Design review of the part built by this model. Coordinates are the model's own, in mm. Face numbers are marked on the shaded views. A direction names the side the tool comes from. Round coordinates to 2 decimals unless told otherwise and drop trailing zeros. Write each loop counter-clockwise with the first axis right and the second up, starting at its lowest first coordinate (ties: lowest second). Pieces come first, ordered by that corner, then holes. Notation, with made-up numbers: (-24.75, 27.25) -> (32.25, 27.25) arc R14 cw to (32.25, 50.25) -> close; hole circle Ø3 at (17, -33.75). An arc over 180 degrees is marked (long way). Write item = value, one per line. Start each with the question number.
Item 1: Machinability: for the marked faces 4 and 5, which of the approach directions +Z, -Z, +X, -X, +Y, -Y give a long, thin tool a straight path to every point of the face, cutting with its end or side? Answer none if there is none.
Item 2: For pin 1 Ø4.5 at (x, y) = (-20, 7) entering from +Z; pin 2 Ø1.2 at (x, z) = (0, 11.5) entering from -Y; pin 3 Ø1.2 at (x, y) = (-20, -6) entering from +Z; pin 4 Ø1.8 at (x, y) = (20.59, 6.89) entering from +Z, all flat-tipped, find the tip position at first contact; note any pin that passes through.
Item 3: Add section D-D, the plane y = -1.25. State the section outline as (x, z) points.
Item 4: Add section C-C, the plane x = -14.5. State the section outline as (y, z) points, then the cut area to 3 significant figures.
Item 5: To check wall thickness, follow L1, parallel to Y at x = -20.59, z = 0.45; L2, parallel to Z at x = 0, y = -14.3 (3 decimals); L3, parallel to Y at x = -17, z = 11.75. State the ranges of each line that lie inside material, in increasing order.
Item 6: Add section A-A, the plane x = -20.59. State the section outline as (y, z) points.
Item 7: Add section B-B, the plane z = 11.1. State the section outline as (x, y) points (3 decimals).
Item 8: Mouldability with a two-part tool opening along X and no side actions: class the marked faces 1, 2 and 3 as released by +X, released by -X, zero draft, split by the parting line, or undercut.
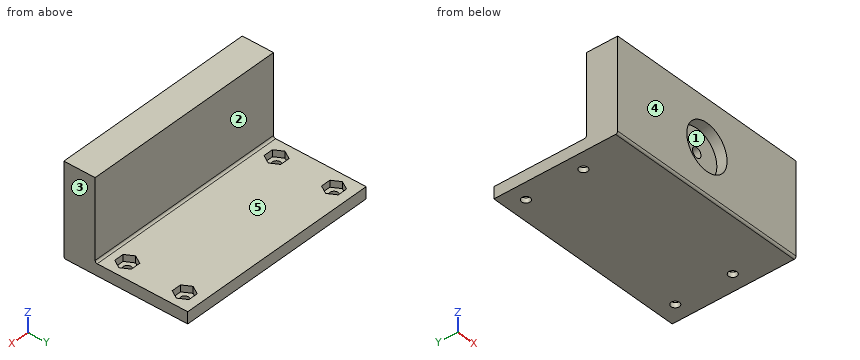
Autodesk Fusion 360 part; units mm, degrees
sketch "Boceto1" plane through (0, 0, 0) normal (0, 0, 1) x (1, 0, 0)
  line L0 (24.6, -11.1) -> (-24.6, -11.1)
  line L1 (-24.6, -11.1) -> (-24.6, 11.1)
  line L2 (-24.6, 11.1) -> (24.6, 11.1)
  line L3 (24.6, 11.1) -> (24.6, -11.1)
  line L4 (24.6, -11.1) -> (-24.6, 11.1) construction
  line L5 (-24.6, -11.1) -> (24.6, 11.1) construction
  circle A0 centre (-20.59, 6.89) radius 1
  line L6 (-24.6, 0) -> (24.6, 0) construction
  circle A1 centre (-20.59, -6.89) radius 1
  line L7 (-20.59, 6.89) -> (-20.59, -6.89) construction
  line L8 (0, 11.1) -> (0, -11.1) construction
  circle A2 centre (20.59, 6.89) radius 1
  circle A3 centre (20.59, -6.89) radius 1
  line L9 (24.6, -18.6) -> (-24.6, -18.6)
  line L10 (-24.6, -18.6) -> (-24.6, -11.1)
  line L11 (-24.6, -11.1) -> (24.6, -11.1)
  line L12 (24.6, -11.1) -> (24.6, -18.6)
  line L13 (24.6, -18.6) -> (-24.6, -11.1) construction
  line L14 (-24.6, -18.6) -> (24.6, -11.1) construction
  point P0 (-20.59, -5.89)
  point P1 (-20.59, 5.89)
  point P2 (0, -14.85)
  dimension "d1" = 22.2
  dimension "d2" = 49.2
  dimension "d3" = 2
  dimension "d4" = 4.01
  dimension "d5" = 4.21
  dimension "d10" = 49.2
  dimension "d11" = 7.5
extrude "Extruir1" add sketch "Boceto1" along normal blind 2.8 contours L0 L1 L2 L3 L11
extrude "Extruir2" add sketch "Boceto1" along normal blind 22.2 contours L0 L9 L10 L11 L12
fillet "Empalme1" radius 0.5 1 edges at (0, -11.1, 2.8)
sketch "Boceto2" plane through (0, -18.6, 0) normal (0, -1, 0) x (1, 0, 0)
  line L0 (-24.6, 0) -> (24.6, 0)
  line L1 (24.6, 0) -> (24.6, 22.2)
  line L2 (24.6, 22.2) -> (-24.6, 22.2)
  line L3 (-24.6, 22.2) -> (-24.6, 0)
  circle A0 centre (0, 11.1) radius 5.55
  line L4 (-24.6, 11.1) -> (24.6, 11.1) construction
  circle A1 centre (0, 11.1) radius 1.175
  dimension "d20" = 11.1
  dimension "d21" = 2.35
extrude "Extruir3" cut sketch "Boceto2" against normal blind 2.45 contours A0
extrude "Extruir4" cut sketch "Boceto2" against normal blind 4.9 contours A1
sketch "Boceto3" plane through (0, 0, 2.8) normal (0, 0, 1) x (-1, 0, 0)
  line L0 (24.6, 10.6) -> (-24.6, 10.6)
  line L1 (-24.6, 10.6) -> (-24.6, -11.1)
  line L2 (-24.6, -11.1) -> (24.6, -11.1)
  line L3 (24.6, -11.1) -> (24.6, 10.6)
  circle A0 centre (-20.59, -6.89) radius 1
  circle A1 centre (20.59, -6.89) radius 1
  circle A2 centre (20.59, 6.89) radius 1
  circle A3 centre (-20.59, 6.89) radius 1
  line L4 (-19.4353, -8.89) -> (-18.2806, -6.89)
  line L5 (-18.2806, -6.89) -> (-19.4353, -4.89)
  line L6 (-19.4353, -4.89) -> (-21.7447, -4.89)
  line L7 (-21.7447, -4.89) -> (-22.8994, -6.89)
  line L8 (-22.8994, -6.89) -> (-21.7447, -8.89)
  line L9 (-21.7447, -8.89) -> (-19.4353, -8.89)
  line L10 (0, 10.6) -> (0, -11.1) construction
  line L11 (-18.2806, 6.89) -> (-19.4353, 8.89)
  line L12 (-19.4353, 8.89) -> (-21.7447, 8.89)
  line L13 (-21.7447, 8.89) -> (-22.8994, 6.89)
  line L14 (-22.8994, 6.89) -> (-21.7447, 4.89)
  line L15 (-21.7447, 4.89) -> (-19.4353, 4.89)
  line L16 (-19.4353, 4.89) -> (-18.2806, 6.89)
  line L17 (21.7447, -8.89) -> (19.4353, -8.89)
  line L18 (19.4353, -8.89) -> (18.2806, -6.89)
  line L19 (18.2806, -6.89) -> (19.4353, -4.89)
  line L20 (22.8994, -6.89) -> (21.7447, -8.89)
  line L21 (21.7447, -4.89) -> (22.8994, -6.89)
  line L22 (19.4353, -4.89) -> (21.7447, -4.89)
  line L23 (21.7447, 4.89) -> (19.4353, 4.89)
  line L24 (19.4353, 4.89) -> (18.2806, 6.89)
  line L25 (18.2806, 6.89) -> (19.4353, 8.89)
  line L26 (19.4353, 8.89) -> (21.7447, 8.89)
  line L27 (21.7447, 8.89) -> (22.8994, 6.89)
  line L28 (22.8994, 6.89) -> (21.7447, 4.89)
  point P0 (-20.59, -6.89)
  point P1 (-20.59, 6.89)
  dimension "d26" = 2
  dimension "d27" = 2
extrude "Extruir5" cut sketch "Boceto3" against normal blind 1.6 contours L4 L5 L6 L7 L8 L9 | L11 L12 L13 L14 L15 L16 | L17 L18 L19 L20 L21 L22 | L23 L24 L25 L26 L27 L28
fillet "Empalme3" radius 0.5 1 edges at (0, -18.6, 0)
equation "d1 = 18 mm + tolerancia * 2 + grosor2 * 2"
equation "d2 = 45 mm + tolerancia * 2 + grosor2 * 2"
equation "d3 = 1.9 mm + tolerancia"
equation "d4 = 1.91 mm + grosor2 + tolerancia"
equation "d5 = 2.11 mm + grosor2 + tolerancia"
equation "grosor1 = 2.8 mm"
equation "grosor2 = 2 mm"
equation "grosor3 = 7.5 mm"
equation "tolerancia = 0.1 mm"
equation "d10 = d2"
equation "d11 = grosor3"
equation "d12 = grosor1"
equation "d14 = d1"
equation "d20 = 11 mm + tolerancia"
equation "d21 = 2.25 mm + tolerancia"
properties part number "Configuracion 1"
Result set:
q1.face_4 = +Z, -Z, +X, -X, -Y
q1.face_5 = +Z, +X, -X, +Y
q2.pin_1 = 2.8
q2.pin_2 = -13.7
q2.pin_3 = 1.2
q2.pin_4 = through
q3.outline = (-24.6, 0) -> (24.6, 0) -> (24.6, 2.8) -> (-24.6, 2.8) -> close
q4.outline = (-18.6, 0.5) arc R0.5 ccw to (-18.1, 0) -> (11.1, 0) -> (11.1, 2.8) -> (-10.6, 2.8) arc R0.5 cw to (-11.1, 3.3) -> (-11.1, 22.2) -> (-18.6, 22.2) -> close
q4.area = 229 mm²
q5.L1 = -18.6 to -7.89, -5.89 to 5.89, 7.89 to 11.1
q5.L2 = 0 to 9.925, 12.275 to 22.2
q5.L3 = -18.6 to -11.1
q6.outline = (-18.6, 0.5) arc R0.5 ccw to (-18.1, 0) -> (-7.89, 0) -> (-7.89, 1.2) -> (-8.89, 1.2) -> (-8.89, 2.8) -> (-10.6, 2.8) arc R0.5 cw to (-11.1, 3.3) -> (-11.1, 22.2) -> (-18.6, 22.2) -> close; (-5.89, 0) -> (5.89, 0) -> (5.89, 1.2) -> (4.89, 1.2) -> (4.89, 2.8) -> (-4.89, 2.8) -> (-4.89, 1.2) -> (-5.89, 1.2) -> close; (7.89, 0) -> (11.1, 0) -> (11.1, 2.8) -> (8.89, 2.8) -> (8.89, 1.2) -> (7.89, 1.2) -> close
q7.outline = (-24.6, -18.6) -> (-5.55, -18.6) -> (-5.55, -16.15) -> (-1.175, -16.15) -> (-1.175, -13.7) -> (1.175, -13.7) -> (1.175, -16.15) -> (5.55, -16.15) -> (5.55, -18.6) -> (24.6, -18.6) -> (24.6, -11.1) -> (-24.6, -11.1) -> close
q8.face_1 = undercut
q8.face_2 = zero draft
q8.face_3 = released by +X
